Can you work these out from the model? Positions are in its coordinate system, mm. A direction names the side the tool comes from. Coordinates: 2 decimals unless noted, no trailing zeros. Write each loop counter-clockwise with the first axis right and the second up, starting at its lowest first coordinate (ties: lowest second). Pieces come first, ordered by that corner, then holes. Notation, with made-up numbers: (86, -11.75) -> (127, -11.75) arc R14 ccw to (127, -4.75) -> close; hole circle Ø3 at (29, 17). An arc over 180 degrees is marked (long way). Use one line per item in the form item = value.
```python
from build123d import *

# Parameters (mm, degrees)
F1_DEPTH = 16
F2_W     = 20
F2_H     = 3.5
F3_DEPTH = 5
F5_DEPTH = 5
F6_W     = 17.5
F6_H     = 1.3
F7_DEPTH = 8
F8_R     = 0.5


# Not quite as in the source:
# - ends of sketch curves that miss each other by under 0.0002 mm in the source are joined


with BuildPart() as f1:
    # F0 (on Right) → F1 (new body)
    with BuildSketch(Plane.YZ):
        Polygon((14.15, 1.3), (14.15, 2.5), (3.35, 2.5), (3.35, 1.3), (0, 1.3), (0, 0), (17.5, 0), (17.5, 1.3), align=None)
    extrude(amount=F1_DEPTH)

    # F2 (on face) → F3 (join)
    with BuildSketch(Plane(origin=(0, 0, 0), x_dir=(0, -1, 0), z_dir=(-1, 0, 0))):
        with Locations((-8.75, 0.75)):
            Rectangle(F2_W, F2_H)
    extrude(amount=F3_DEPTH)

    # F4 (on face) → F5 (cut)
    with BuildSketch(Plane.XY.offset(2.5)):
        with BuildLine():
            ThreePointArc((16.0075383861, 14.2499948339), (10.5000136527, 8.7377452223), (16.0320477827, 3.2500933699))
            Line((16.0320477827, 3.2500933699), (16.0075383861, 14.2499948339))
        make_face()
    extrude(amount=-F5_DEPTH, mode=Mode.SUBTRACT)

    # F6 (on face) → F7 (cut)
    with BuildSketch(Plane.YZ.offset(16)):
        with Locations((8.75, 0.65)):
            Rectangle(F6_W, F6_H)
    extrude(amount=-F7_DEPTH, mode=Mode.SUBTRACT)

    # F8
    f8_edges = [f1.edges().sort_by_distance(p)[0] for p in [
        (7.477985, 3.35, 2.5),
        (14.955969, 3.35, 1.9),
        (14.955969, 14.15, 1.9),
        (10.5, 8.75, 2.5),
        (10.5, 8.75, 1.3),
        (7.477985, 14.15, 2.5),
        (8, 8.75, 1.3),
        (0, 8.75, 0),
        (0, 1.675, 1.3),
        (0, 0, 0.65),
        (0, 17.5, 0.65),
        (0, 15.825, 1.3),
        (-5, 8.75, -1),
        (-5, -1.25, 0.75),
        (-5, 8.75, 2.5),
        (-5, 18.75, 0.75),
        (-2.5, -1.25, -1),
        (-2.5, -1.25, 2.5),
        (0, -1.25, 0.75),
        (-2.5, 18.75, 2.5),
        (-2.5, 18.75, -1),
        (0, 18.75, 0.75),
        (4, 17.5, 1.3),
        (8, 17.5, 0.65),
        (4, 17.5, 0),
        (4, 0, 0),
        (8, 0, 0.65),
        (4, 0, 1.3),
        (8, 8.75, 0),
        (0, 1.05, 2.5),
        (0, 16.45, 2.5),
        (0, 3.35, 1.9),
        (0, 14.15, 1.9),
    ]]
    fillet(f8_edges, radius=F8_R)


solid = f1.part
```
Q1. Suppose I cut it at B-B (x = 2.75). Write out the boundary of the cut face in (y, z).
Return value:
outline = (0, 0.5) arc R0.5 ccw to (0.5, 0) -> (17, 0) arc R0.5 ccw to (17.5, 0.5) -> (17.5, 0.8) arc R0.5 ccw to (17, 1.3) -> (14.15, 1.3) -> (14.15, 2) arc R0.5 ccw to (13.65, 2.5) -> (3.85, 2.5) arc R0.5 ccw to (3.35, 2) -> (3.35, 1.3) -> (0.5, 1.3) arc R0.5 ccw to (0, 0.8) -> close
Q2. Suppose I cut it at C-C (x = 9). Write out the boundary of the cut face in (y, z).
Return value:
outline = (3.35, 1.3) -> (14.15, 1.3) -> (14.15, 2) arc R0.5 ccw to (13.65, 2.5) -> (3.85, 2.5) arc R0.5 ccw to (3.35, 2) -> close
Q3. Thinking about a two-plate mould opening in Y: for faces 1 (the flat face through (4, 9, 0)), 2 (the flat face through (-2, -1.25, 1)), 3 (the flat face through (-2, 18.75, 1)), which applies, released by +Y, released by -Y, zero draft, split by the parting line, or undercut?
Return value:
face_1 = zero draft
face_2 = released by -Y
face_3 = released by +Y
Q4. Will these pins go through, and if not, where does the flat tip stop? pin 1 (5.5 mm diameter, centred on x = 3.5, y = 11.5, fed in from -Z); pin 2 (0.9 mm diameter, centred on y = 12.5, z = 0, fed in from +X); pin 3 (3 mm diameter, centred on x = 4, y = 16, fed in from +Z).
Return value:
pin_1 = 0
pin_2 = 8
pin_3 = 1.3
Q5. Suppose I cut it at A-A (y = 2). Write out the boundary of the cut face in (x, z).
Return value:
outline = (-5, -0.5) arc R0.5 ccw to (-4.5, -1) -> (0, -1) -> (0, -0.5) arc R0.5 cw to (0.5, 0) -> (7.5, 0) arc R0.5 ccw to (8, 0.5) -> (8, 1.3) -> (0.5, 1.3) arc R0.5 cw to (0, 1.8) -> (0, 2) arc R0.5 ccw to (-0.5, 2.5) -> (-4.5, 2.5) arc R0.5 ccw to (-5, 2) -> close
Q6. If I drill on line 1 (Z direction, x = 1, y = 8); line 2 (X direction, y = 2, z = 1.05); line 3 (Z direction, x = 4.75, y = 16.5), over which ranges is the centre line in solid material (lowest first)? Write a range as from..to.
Return value:
line_1 = 0..2.5
line_2 = -5..8
line_3 = 0..1.3
Q7. For faces 4 (the flat face through (4, 2, 1.3)), 5 (the flat face through (9.8, 8.7, 1.3)), 6 (the flat face through (4, 16, 1.3)), which set-ups out of +Z, -Z, +X, -X, +Y, -Y let a thin tool reach every point of the face, with its end or its side?
Return value:
face_4 = +Z, +X, -Y
face_5 = -Z, +X, +Y, -Y
face_6 = +Z, +X, +Y
